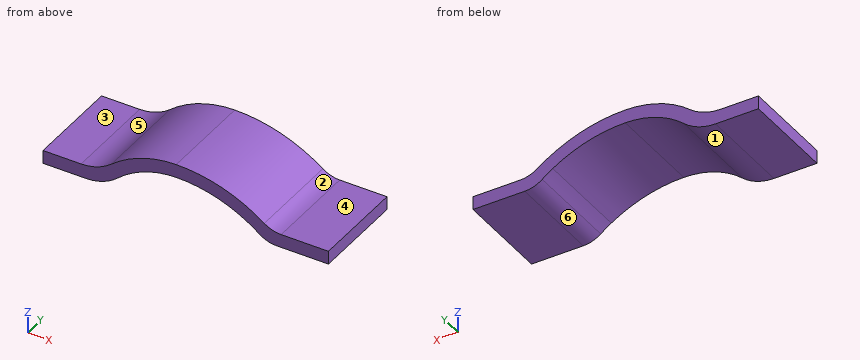
```python
from build123d import *

# Parameters (mm, degrees)
F6_DEPTH  = 25
F7_DEPTH  = 25
F8_DEPTH  = 25
F9_DEPTH  = 25
F10_DEPTH = 25
F11_R     = 25
F12_R     = 15


with BuildPart() as f6:
    # F3 (on Front) → F6 (new body, symmetric)
    with BuildSketch(Plane.XZ):
        Polygon((-70, 0), (0, 0), (80, 0), (80, 7), (50, 7), (-40, 7), (-70, 7), align=None)
    extrude(amount=F6_DEPTH, both=True)

    # F4 (on Front) → F7 (join, symmetric)
    with BuildSketch(Plane.XZ):
        with BuildLine():
            Line((0, 18), (0, 25))
            ThreePointArc((0, 25), (-25.8467706988, 18.3343230299), (-45.2462398683, 0))
            Line((-45.2462398683, 0), (-36.7151195014, 0))
            ThreePointArc((-36.7151195014, 0), (-20.4450483003, 13.257910642), (0, 18))
        make_face()
    extrude(amount=F7_DEPTH, both=True)

    # F5 (on Front) → F8 (join, symmetric)
    with BuildSketch(Plane.XZ):
        with BuildLine():
            Line((47.4130783645, 0), (57.4214439232, 0))
            ThreePointArc((57.4214439232, 0), (31.3138237134, 18.4789544508), (0, 25))
            Line((0, 25), (0, 18))
            ThreePointArc((0, 18), (25.3574446662, 13.3485839491), (47.4130783645, 0))
        make_face()
    extrude(amount=F8_DEPTH, both=True)

    # F4 (on Front) → F9 (cut, symmetric)
    with BuildSketch(Plane.XZ):
        with BuildLine():
            Line((0, 0), (0, 18))
            ThreePointArc((0, 18), (-20.4450483003, 13.257910642), (-36.7151195014, 0))
            Line((-36.7151195014, 0), (0, 0))
        make_face()
        with BuildLine():
            Line((0, 0), (-36.7151195014, 0))
            ThreePointArc((-36.7151195014, 0), (-41.7023550864, -48.8894927447), (0, -74.8888888889))
            Line((0, -74.8888888889), (0, 0))
        make_face()
    extrude(amount=F9_DEPTH, both=True, mode=Mode.SUBTRACT)

    # F5 (on Front) → F10 (cut, symmetric)
    with BuildSketch(Plane.XZ):
        with BuildLine():
            Line((0, 0), (0, -124.8888888889))
            ThreePointArc((0, -124.8888888889), (66.7930283935, -78.8018891107), (47.4130783645, 0))
            Line((47.4130783645, 0), (0, 0))
        make_face()
        with BuildLine():
            Line((0, 0), (47.4130783645, 0))
            ThreePointArc((47.4130783645, 0), (25.3574446662, 13.3485839491), (0, 18))
            Line((0, 18), (0, 0))
        make_face()
    extrude(amount=F10_DEPTH, both=True, mode=Mode.SUBTRACT)

    # F11
    f11_edges = [f6.edges().sort_by_distance(p)[0] for p in [
        (-40, 0, 7),
        (-36.71512, 0, 0),
    ]]
    fillet(f11_edges, radius=F11_R)

    # F12
    f12_edges = [f6.edges().sort_by_distance(p)[0] for p in [
        (50, 0, 7),
        (47.413078, 0, 0),
    ]]
    fillet(f12_edges, radius=F12_R)


solid = f6.part
```
The listing builds one solid part. Answer for the finished solid, in the listing's coordinates (mm). Face numbers are marked on the shaded views. A direction names the side the tool comes from. Give positions to 0.01 mm unless a question says otherwise; leave off trailing zeros. Order: outer loops, then holes, each group sorted by start corner. A loop starts at its lowest first (then second) coordinate and runs counter-clockwise, first axis right, second up. Notation, with made-up numbers: (-35.75, 70.5) - (17.25, 70.5) arc R10 cw to (17.25, 82.5) - close; hole circle Ø2 at (13.5, 83). An arc over 180 degrees is marked (long way). Answer in a Markdown table with one row per item. Add a question column.
Q1. Given P1, Ø16, axis at x = -56, y = -11, coming from the +Z side; P2, Ø12.5, axis at x = 64.5, y = -11.5, coming from the +Z side; P3, Ø1.5, axis at y = -18.5, z = 19, coming from the +X side; P4, Ø4, axis at x = -39.5, z = 13.5, coming from the -Y side, each flat-ended and moving along its own axis, determine where each tip first touches the part or whether it passes through.
Q2. The part is cut by section B-B (y = 13). Determine the outline of the cut face in (x, z).
Q3. The part is cut by section D-D (z = 23). Determine the outline of the cut face in (x, y), then the cut area to 3 significant figures.
Q4. The part is cut by section A-A (z = 14.5). Determine the outline of the cut face in (x, y), then the cut area to 3 significant figures.
Q5. For a pull along X with two mould halves and no side action, classify the marked faces 4, 5 and 6 as released by +X, released by -X, zero draft, split by the parting line, or undercut.
Q6. Find the intervals of material crossed by line 1 along Z through (x, y) = (-52, -15.5); line 2 along X through (y, z) = (10.5, 4); line 3 along Z through (x, y) = (-1.5, 14), in increasing order. Write a range as [from, to].
Q7. Which of the six approach directions +Z, -Z, +X, -X, +Y, -Y give full straight-line access (tool end or side, diameter ignored) to the marked faces 1, 2 and 3?
Q8. The part is cut by section C-C (x = 68.5). Determine the outline of the cut face in (y, z).
Determined:
| question | item | result |
|---|---|---|
| 1 | P1 | stops at z = 7.08 |
| 1 | P2 | stops at z = 7 |
| 1 | P3 | stops at x = 31.83 |
| 1 | P4 | passes through |
| 2 | outline | (-70, 0) - (-47.41, 0) arc R25 ccw to (-30.82, 6.3) arc R46.44 cw to (0, 18) arc R71.44 cw to (43.64, 3.12) arc R15 ccw to (52.8, 0) - (80, 0) - (80, 7) - (55.14, 7) arc R15 cw to (46.29, 9.89) arc R78.44 ccw to (0, 25) arc R53.44 ccw to (-34.07, 12.74) arc R25 cw to (-50, 7) - (-70, 7) - close |
| 3 | outline | (-14.48, -25) - (17.6, -25) - (17.6, 25) - (-14.48, 25) - close |
| 3 | area | 1,600 mm² |
| 4 | outline | (-31.81, -25) - (-17.69, -25) - (-17.69, 25) - (-31.81, 25) - close; (22.09, -25) - (39.21, -25) - (39.21, 25) - (22.09, 25) - close |
| 4 | area | 1,560 mm² |
| 5 | face 4 | zero draft |
| 5 | face 5 | released by -X |
| 5 | face 6 | undercut |
| 6 | line 1 | z = [0, 7] |
| 6 | line 2 | x = [-70, -33.85], [42.48, 80] |
| 6 | line 3 | z = [17.98, 24.98] |
| 7 | face 1 | -Z, +Y, -Y |
| 7 | face 2 | +Z, +X, +Y, -Y |
| 7 | face 3 | +Z, -X, +Y, -Y |
| 8 | outline | (-25, 0) - (25, 0) - (25, 7) - (-25, 7) - close |
